Read the model definition and answer for the solid it produces. Units are mm, in the model's axes. A direction names the side the tool comes from. Coordinates: 2 decimals unless noted, no trailing zeros. Loops run counter-clockwise (first coordinate to the right, second up) from the corner with the lowest first, then second, coordinate; pieces in that order, holes last.
from build123d import *

# Parameters (mm, degrees)
F0_W          = 26.8
F0_H          = 47
F1_DEPTH      = 18
F2_SIZE       = 6
F3_R          = 2
F5_DEPTH      = 5
F6_R          = 1
F7_W          = 28.5
F7_H          = 54.5
F8_DEPTH      = 3
F10_R         = 1.75
F11_DEPTH     = 1.8
F12_T4_DEPTH  = 13
F12_T9_DEPTH  = 13
F12_T14_DEPTH = 13
F12_T19_DEPTH = 13
F12_T24_DEPTH = 13
F12_T29_DEPTH = 13
F12_T34_DEPTH = 13
F12_T39_DEPTH = 13
F13_R         = 1
F14_SIZE      = 1.3
F15_W         = 24
F15_H         = 16.5
F16_DEPTH     = 10
F17_SIZE      = 6
F19_R         = 2
F20_R         = 0.5
F21_W         = 16
F21_H         = 10.5
F22_DEPTH     = 10
F24_DEPTH     = 10.5
F25_R         = 0.5


# Not quite as in the source:
# - a fillet or chamfer that OpenCascade refuses, or shapes differently, is made with other operations: its cross-section is extruded or revolved along the edge and cut away or added


with BuildPart() as f1:
    # F0 (on Front) → F1 (new body)
    with BuildSketch(Plane.XZ):
        Rectangle(F0_W, F0_H)
    extrude(amount=-F1_DEPTH)

    # F2
    f2_edges = [f1.edges().sort_by_distance(p)[0] for p in [
        (-13.4, 9, 23.5),
        (13.4, 9, 23.5),
    ]]
    chamfer(f2_edges, length=F2_SIZE)

    # F3
    f3_edges = [f1.edges().sort_by_distance(p)[0] for p in [
        (-13.4, 9, -23.5),
        (13.4, 9, -23.5),
    ]]
    fillet(f3_edges, radius=F3_R)

    # F4 (on face) → F5 (cut)
    with BuildSketch(Plane(origin=(0, 18, 0), x_dir=(-1, 0, 0), z_dir=(0, 1, 0))):
        Polygon((-6.5715728753, 21.5), (-11.4, 16.6715728753), (-11.4, -21.5), (11.4, -21.5), (11.4, 16.6715728753), (6.5715728753, 21.5), align=None)
    extrude(amount=-F5_DEPTH, mode=Mode.SUBTRACT)

    # F6
    f6_edges = [f1.edges().sort_by_distance(p)[0] for p in [
        (-11.4, 15.5, -21.5),
        (-11.4, 15.5, 16.671573),
        (-6.571573, 15.5, 21.5),
        (6.571573, 15.5, 21.5),
        (11.4, 15.5, 16.671573),
        (11.4, 15.5, -21.5),
        (-8.985786, 13, 19.085786),
        (0, 13, 21.5),
        (8.985786, 13, 19.085786),
        (11.4, 13, -2.414214),
        (0, 13, -21.5),
        (-11.4, 13, -2.414214),
    ]]
    fillet(f6_edges, radius=F6_R)

    # F7 (on face) → F8 (join)
    with BuildSketch(Plane.XZ):
        Rectangle(F7_W, F7_H)
    extrude(amount=F8_DEPTH)

    # F10 (on offset) → F11 (join)
    with BuildSketch(Plane.XZ.offset(1.8)):
        Polygon((24.35, 0), (13.25, 29.25), (-13.25, 29.25), (-24.35, 0), (-13.25, -29.25), (13.25, -29.25), align=None)
        with Locations((-20, 0)):
            Circle(F10_R, mode=Mode.SUBTRACT)
        with Locations((20, 0)):
            Circle(F10_R, mode=Mode.SUBTRACT)
    extrude(amount=-F11_DEPTH)

    # F12: fillet of radius 2 on 4 edges, made by hand


with BuildPart() as f12_tool2:
    # F12_s3 → F12_t4 (new body)
    with BuildSketch(Plane.XZ.offset(-5)):
        with BuildLine():
            ThreePointArc((12.25, 27.25), (13.6642135624, 26.6642135624), (14.25, 25.25))
            Line((14.25, 25.25), (14.25, 27.25))
            Line((14.25, 27.25), (12.25, 27.25))
        make_face()
    extrude(amount=F12_T4_DEPTH)

    split(bisect_by=Plane.XZ.offset(1.8), keep=Keep.TOP)


with BuildPart() as f1_1:
    add(f1.part)

    # F12_t1: cut F12_tool2
    add(f12_tool2.part, mode=Mode.SUBTRACT)


with BuildPart() as f12_tool7:
    # F12_s8 → F12_t9 (new body)
    with BuildSketch(Plane.XZ.offset(-5)):
        with BuildLine():
            ThreePointArc((12.25, 27.25), (13.6642135624, 26.6642135624), (14.25, 25.25))
            Line((14.25, 25.25), (14.25, 27.25))
            Line((14.25, 27.25), (12.25, 27.25))
        make_face()
    extrude(amount=F12_T9_DEPTH)

    split(bisect_by=Plane(origin=(21.2847693156, 0, 8.0772970736), x_dir=(0, 1, 0), z_dir=(0.9349426915, 0, 0.354798765)), keep=Keep.TOP)


with BuildPart() as f1_2:
    add(f1_1.part)

    # F12_t6: cut F12_tool7
    add(f12_tool7.part, mode=Mode.SUBTRACT)


with BuildPart() as f12_tool12:
    # F12_s13 → F12_t14 (new body)
    with BuildSketch(Plane.XZ.offset(-5)):
        with BuildLine():
            ThreePointArc((-12.25, 27.25), (-13.6642135624, 26.6642135624), (-14.25, 25.25))
            Line((-14.25, 25.25), (-14.25, 27.25))
            Line((-14.25, 27.25), (-12.25, 27.25))
        make_face()
    extrude(amount=F12_T14_DEPTH)

    split(bisect_by=Plane.XZ.offset(1.8), keep=Keep.TOP)


with BuildPart() as f1_3:
    add(f1_2.part)

    # F12_t11: cut F12_tool12
    add(f12_tool12.part, mode=Mode.SUBTRACT)


with BuildPart() as f12_tool17:
    # F12_s18 → F12_t19 (new body)
    with BuildSketch(Plane.XZ.offset(-5)):
        with BuildLine():
            ThreePointArc((-12.25, 27.25), (-13.6642135624, 26.6642135624), (-14.25, 25.25))
            Line((-14.25, 25.25), (-14.25, 27.25))
            Line((-14.25, 27.25), (-12.25, 27.25))
        make_face()
    extrude(amount=F12_T19_DEPTH)

    split(bisect_by=Plane(origin=(-21.2847693156, 0, 8.0772970736), x_dir=(0, 1, 0), z_dir=(-0.9349426915, 0, 0.354798765)), keep=Keep.TOP)


with BuildPart() as f1_4:
    add(f1_3.part)

    # F12_t16: cut F12_tool17
    add(f12_tool17.part, mode=Mode.SUBTRACT)


with BuildPart() as f12_tool22:
    # F12_s23 → F12_t24 (new body)
    with BuildSketch(Plane.XZ.offset(-5)):
        with BuildLine():
            ThreePointArc((14.25, -25.25), (13.6642135624, -26.6642135624), (12.25, -27.25))
            Line((12.25, -27.25), (14.25, -27.25))
            Line((14.25, -27.25), (14.25, -25.25))
        make_face()
    extrude(amount=F12_T24_DEPTH)

    split(bisect_by=Plane.XZ.offset(1.8), keep=Keep.TOP)


with BuildPart() as f1_5:
    add(f1_4.part)

    # F12_t21: cut F12_tool22
    add(f12_tool22.part, mode=Mode.SUBTRACT)


with BuildPart() as f12_tool27:
    # F12_s28 → F12_t29 (new body)
    with BuildSketch(Plane.XZ.offset(-5)):
        with BuildLine():
            ThreePointArc((14.25, -25.25), (13.6642135624, -26.6642135624), (12.25, -27.25))
            Line((12.25, -27.25), (14.25, -27.25))
            Line((14.25, -27.25), (14.25, -25.25))
        make_face()
    extrude(amount=F12_T29_DEPTH)

    split(bisect_by=Plane(origin=(21.2847693156, 0, -8.0772970736), x_dir=(0, 1, 0), z_dir=(0.9349426915, 0, -0.354798765)), keep=Keep.TOP)


with BuildPart() as f1_6:
    add(f1_5.part)

    # F12_t26: cut F12_tool27
    add(f12_tool27.part, mode=Mode.SUBTRACT)


with BuildPart() as f12_tool32:
    # F12_s33 → F12_t34 (new body)
    with BuildSketch(Plane.XZ.offset(-5)):
        with BuildLine():
            ThreePointArc((-14.25, -25.25), (-13.6642135624, -26.6642135624), (-12.25, -27.25))
            Line((-12.25, -27.25), (-14.25, -27.25))
            Line((-14.25, -27.25), (-14.25, -25.25))
        make_face()
    extrude(amount=F12_T34_DEPTH)

    split(bisect_by=Plane.XZ.offset(1.8), keep=Keep.TOP)


with BuildPart() as f1_7:
    add(f1_6.part)

    # F12_t31: cut F12_tool32
    add(f12_tool32.part, mode=Mode.SUBTRACT)


with BuildPart() as f12_tool37:
    # F12_s38 → F12_t39 (new body)
    with BuildSketch(Plane.XZ.offset(-5)):
        with BuildLine():
            ThreePointArc((-14.25, -25.25), (-13.6642135624, -26.6642135624), (-12.25, -27.25))
            Line((-12.25, -27.25), (-14.25, -27.25))
            Line((-14.25, -27.25), (-14.25, -25.25))
        make_face()
    extrude(amount=F12_T39_DEPTH)

    split(bisect_by=Plane(origin=(-21.2847693156, 0, -8.0772970736), x_dir=(0, 1, 0), z_dir=(-0.9349426915, 0, -0.354798765)), keep=Keep.TOP)


with BuildPart() as f1_8:
    add(f1_7.part)

    # F12_t36: cut F12_tool37
    add(f12_tool37.part, mode=Mode.SUBTRACT)

    # F13
    f13_edges = [f1_8.edges().sort_by_distance(p)[0] for p in [
        (-13.25, -0.9, 29.25),
        (13.25, -0.9, 29.25),
        (-24.35, -0.9, 0),
        (-13.25, -0.9, -29.25),
        (13.25, -0.9, -29.25),
        (24.35, -0.9, 0),
    ]]
    fillet(f13_edges, radius=F13_R)

    # F14
    f14_edges = [f1_8.edges().sort_by_distance(p)[0] for p in [
        (-21.75, -1.8, 0),
        (18.25, -1.8, 0),
    ]]
    chamfer(f14_edges, length=F14_SIZE)


with BuildPart() as f16:
    # F15 (on face) → F16 (new body)
    with BuildSketch(Plane.XZ.offset(3)):
        with Locations((0, 15)):
            Rectangle(F15_W, F15_H)
    extrude(amount=-F16_DEPTH)

    # F17
    f17_edges = [f16.edges().sort_by_distance(p)[0] for p in [
        (12, 2, 23.25),
        (-12, 2, 23.25),
    ]]
    chamfer(f17_edges, length=F17_SIZE)


with BuildPart() as f1_9:
    add(f1_8.part)

    # F18: cut F16
    add(f16.part, mode=Mode.SUBTRACT)

    # F19
    f19_edges = [f1_9.edges().sort_by_distance(p)[0] for p in [
        (-12, 2, 6.75),
        (12, 2, 6.75),
    ]]
    fillet(f19_edges, radius=F19_R)

    # F20
    f20_edges = [f1_9.edges().sort_by_distance(p)[0] for p in [
        (12, 2, 17.25),
        (6, 2, 23.25),
        (-12, 2, 17.25),
        (-6, 2, 23.25),
        (12, 7, 13),
        (11.414214, 7, 7.335786),
        (9, 7, 20.25),
        (0, 7, 6.75),
        (0, 7, 23.25),
        (-11.414214, 7, 7.335786),
        (-9, 7, 20.25),
        (-12, 7, 13),
    ]]
    fillet(f20_edges, radius=F20_R)

    # F21 (on face) → F22 (cut)
    with BuildSketch(Plane.XZ.offset(3)):
        with Locations((0, -13.7)):
            Rectangle(F21_W, F21_H)
    extrude(amount=-F22_DEPTH, mode=Mode.SUBTRACT)

    # F23 (on face) → F24 (join, through all)
    with BuildSketch(Plane.XY.offset(-18.95)):
        with BuildLine():
            ThreePointArc((-4.6646603483, -9.9856908622), (0.7682384829, -4.8622275452), (8, -3))
            Line((8, -3), (8, -1.4239461161))
            Line((8, -1.4239461161), (-8, -1.4239461161))
            Line((-8, -1.4239461161), (-8, -3))
            ThreePointArc((-8, -3), (-7.1233945241, -6.8705415453), (-4.6646603483, -9.9856908622))
        make_face()
    extrude(amount=F24_DEPTH)

    # F25
    f25_edges = [f1_9.edges().sort_by_distance(p)[0] for p in [
        (-4.66466, -9.985691, -13.7),
    ]]
    fillet(f25_edges, radius=F25_R)


solid = f1_9.part
Item 1: A cutting plane is placed at D-D on y = 8.75. Determine the outline of the cut face in (x, z), then the cut area to 3 significant figures.
Numbers:
outline: (-13.4, -21.5) arc R2 ccw to (-11.4, -23.5) - (11.4, -23.5) arc R2 ccw to (13.4, -21.5) - (13.4, 17.5) - (7.4, 23.5) - (-7.4, 23.5) - (-13.4, 17.5) - close
area: 1,220 mm2
Item 2: A cutting plane is placed at C-C on x = 20. Determine the outline of the cut face in (y, z).
Numbers:
outline: (-1.8, -11.46) - (0, -11.46) - (0, -1.75) - (-0.5, -1.75) - (-1.8, -3.05) - close; (-1.8, 3.05) - (-0.5, 1.75) - (0, 1.75) - (0, 11.46) - (-1.8, 11.46) - close
Item 3: Determine the mould class of faces 1 (the face through (13.65, -2.39, 26.68)), 2 (the face through (0, -1, 29.25)), 3 (the face through (0, 13, 0)) for opening direction X: released by +X, released by -X, zero draft, split by the parting line, or undercut.
Numbers:
face 1: released by +X
face 2: zero draft
face 3: undercut
Item 4: Find the intervals of material crossed by line 1 along Z through (x, y) = (1.5, 1); line 2 along Z through (x, y) = (6.5, -1); line 3 along Y through (x, z) = (15.5, 21), in increasing order.
Numbers:
line 1: z = -23.5 to -18.95, -8.45 to 6.75, 23.25 to 23.5
line 2: z = -29.25 to -18.95, -8.45 to 6.75, 22.75 to 29.25
line 3: y = -1.8 to 0
Item 5: A cutting plane is placed at A-A on y = 3.75. Determine the outline of the cut face in (x, z).
Numbers:
outline: (-13.4, -21.5) arc R2 ccw to (-11.4, -23.5) - (11.4, -23.5) arc R2 ccw to (13.4, -21.5) - (13.4, 17.5) - (7.4, 23.5) - (-7.4, 23.5) - (-13.4, 17.5) - close; hole (-12, 8.75) arc R2 ccw to (-10, 6.75) - (10, 6.75) arc R2 ccw to (12, 8.75) - (12, 17.04) arc R0.5 ccw to (11.85, 17.4) - (6.15, 23.1) arc R0.5 ccw to (5.79, 23.25) - (-5.79, 23.25) arc R0.5 ccw to (-6.15, 23.1) - (-11.85, 17.4) arc R0.5 ccw to (-12, 17.04) - close; hole (-8, -18.95) - (8, -18.95) - (8, -8.45) - (-8, -8.45) - close
Item 6: Which of the six approach directions +Z, -Z, +X, -X, +Y, -Y give full straight-line access (tool end or side, diameter ignored) to faces 4 (the face through (10.4, 8.9, 20.5)), 5 (the face through (8.956, 16.028, 19.115)), 6 (the face through (-10.4, 8.9, 20.5))?
Numbers:
face 4: +Z, +X, +Y
face 5: +Y
face 6: +Z, -X, +Y
Item 7: Given pin 1 (9 mm diameter, centred on x = -5.5, y = 10, fed in from -Z); pin 2 (1 mm diameter, centred on x = 15, y = 13, fed in from +Z); pin 3 (3.5 mm diameter, centred on x = -3, y = -6, fed in from -Z); pin 4 (2.5 mm diameter, centred on y = -0.5, z = 11, fed in from -X), each flat-ended and moving along its own axis, determine where each tip first touches the part or whether it passes through.
Numbers:
pin 1: stops at z = -23.5
pin 2: passes through
pin 3: stops at z = -18.95
pin 4: stops at x = -20.65
